```python
from build123d import *

# Parameters (mm, degrees)
CROQUIS1_R                = 1.5
SALIENTE_EXTRUIR1_DEPTH   = 10
SALIENTE_EXTRUIR1_2_DEPTH = 10
CROQUIS2_W                = 22.2
CROQUIS2_H                = 12
SALIENTE_EXTRUIR2_DEPTH   = 17.8
CROQUIS3_R                = 2.25
SALIENTE_EXTRUIR3_DEPTH   = 3
CROQUIS4_W                = 14.9
CROQUIS4_H                = 6.9
SALIENTE_EXTRUIR4_DEPTH   = 10
CROQUIS5_W                = 12.9
CROQUIS5_H                = 4.9
CROQUIS5_W_2              = 10.8
CROQUIS5_H_2              = 1.83
CORTAR_EXTRUIR1_DEPTH     = 10.5


with BuildPart() as part:
    # Croquis1 → Saliente-Extruir1 (new body)
    with BuildSketch(Plane.XY):
        with BuildLine():
            Line((-9.1, 6), (-9.1, -6))
            Line((-9.1, -6), (-13.25, -6))
            ThreePointArc((-13.25, -6), (-19.25, 0), (-13.25, 6))
            Line((-13.25, 6), (-9.1, 6))
        make_face()
        with Locations((-14.45, 0)):
            Circle(CROQUIS1_R, mode=Mode.SUBTRACT)
    extrude(amount=SALIENTE_EXTRUIR1_DEPTH)



with BuildPart() as body_2:
    # Croquis1 → Saliente-Extruir1 2 (new body)
    with BuildSketch(Plane.XY):
        with BuildLine():
            Line((9.1, 6), (9.1, -6))
            Line((9.1, -6), (13.25, -6))
            ThreePointArc((13.25, -6), (19.25, 0), (13.25, 6))
            Line((13.25, 6), (9.1, 6))
        make_face()
        with Locations((14.45, 0)):
            Circle(CROQUIS1_R, mode=Mode.SUBTRACT)
    extrude(amount=SALIENTE_EXTRUIR1_2_DEPTH)


with BuildPart() as part_1:
    add(part.part)

    add(body_2.part)  # Saliente-Extruir2 merges body 2
    # Croquis2 → Saliente-Extruir2 (add)
    with BuildSketch(Plane.XY.offset(10)):
        Rectangle(CROQUIS2_W, CROQUIS2_H)
    extrude(amount=SALIENTE_EXTRUIR2_DEPTH)

    # Croquis3 → Saliente-Extruir3 (add)
    with BuildSketch(Plane.XY.offset(27.8)):
        Circle(CROQUIS3_R)
    extrude(amount=SALIENTE_EXTRUIR3_DEPTH)

    # Croquis4 → Saliente-Extruir4 (add)
    with BuildSketch(Plane(origin=(0, 0, 10), x_dir=(-1, 0, 0), z_dir=(0, 0, -1))):
        Rectangle(CROQUIS4_W, CROQUIS4_H)
    extrude(amount=SALIENTE_EXTRUIR4_DEPTH)

    # Croquis5 → Cortar-Extruir1 (cut)
    with BuildSketch(Plane(origin=(0, 0, 0), x_dir=(-1, 0, 0), z_dir=(0, 0, -1))):
        Rectangle(CROQUIS5_W, CROQUIS5_H)
        with Locations((0, 0.915)):
            Rectangle(CROQUIS5_W_2, CROQUIS5_H_2, mode=Mode.SUBTRACT)
    extrude(amount=-CORTAR_EXTRUIR1_DEPTH, mode=Mode.SUBTRACT)


solid = part_1.part
```
Check sheet for the modelled part. Datum: model origin and axes. Units: mm. A direction names the side the tool comes from. Round coordinates to 2 decimals unless told otherwise and drop trailing zeros. Write each loop counter-clockwise with the first axis right and the second up, starting at its lowest first coordinate (ties: lowest second). Pieces come first, ordered by that corner, then holes. Notation, with made-up numbers: (73.5, 61) -> (128.5, 61) arc R13 cw to (128.5, 74) -> close; hole circle Ø3 at (87.25, 2). An arc over 180 degrees is marked (long way). Put each result on its own line as item: value.
(1) Material ranges on line 1 (Y direction, x = -5, z = 6); line 2 (X direction, y = -1.25, z = 8); line 3 (Z direction, x = -12.5, y = -0.5), recorded low to high.
Values found:
line 1: y = -3.45 to -2.45, 0 to 1.83, 2.45 to 3.45
line 2: x = -19.12 to -15.28, -13.62 to -9.1, -7.45 to -6.45, 6.45 to 7.45, 9.1 to 13.62, 15.28 to 19.12
line 3: z = 0 to 10
(2) Tool access check on faces 1 (the face through (-13, -1, 10)), 2 (the face through (0, 0, 30.8)), 3 (the face through (0, 1, 0)), 4 (the face through (0, 0, 5)), 5 (the face through (-9.1, 0, 5)). Record the directions out of +Z, -Z, +X, -X, +Y, -Y that give a thin tool (end or side, any length) a straight path to the whole face; none if there is none.
Values found:
face 1: +Z, -X, +Y, -Y
face 2: +Z, +X, -X, +Y, -Y
face 3: -Z, +X, -X, +Y, -Y
face 4: -Z
face 5: -Z, +Y, -Y
(3) Sectioned sample at D-D (x = 0). Enter the section's corners in (y, z).
Values found:
outline: (-6, 10) -> (-3.45, 10) -> (-3.45, 0) -> (-2.45, 0) -> (-2.45, 10.5) -> (0, 10.5) -> (0, 0) -> (1.83, 0) -> (1.83, 10.5) -> (2.45, 10.5) -> (2.45, 0) -> (3.45, 0) -> (3.45, 10) -> (6, 10) -> (6, 27.8) -> (2.25, 27.8) -> (2.25, 30.8) -> (-2.25, 30.8) -> (-2.25, 27.8) -> (-6, 27.8) -> close
(4) Sectioned sample at C-C (y = -3). Enter the section's corners in (x, z), plus the area to 3 significant figures.
Values found:
outline: (-18.45, 0) -> (-9.1, 0) -> (-9.1, 10) -> (-7.45, 10) -> (-7.45, 0) -> (7.45, 0) -> (7.45, 10) -> (9.1, 10) -> (9.1, 0) -> (18.45, 0) -> (18.45, 10) -> (11.1, 10) -> (11.1, 27.8) -> (-11.1, 27.8) -> (-11.1, 10) -> (-18.45, 10) -> close
area: 731 mm^2
(5) Sectioned sample at B-B (x = 14.45). Enter the section's corners in (y, z), plus the area to 3 significant figures.
Values found:
outline: (-5.88, 0) -> (-1.5, 0) -> (-1.5, 10) -> (-5.88, 10) -> close; (1.5, 0) -> (5.88, 0) -> (5.88, 10) -> (1.5, 10) -> close
area: 87.6 mm^2
(6) Mould release check, pull along X, two halves, no side actions. Record for faces 6 (the face through (6.45, 0, 5)), 7 (the face through (19.25, -0.13, 4.93)), 8 (the face through (-0.29, 2.23, 29.28)), 9 (the face through (13, -1, 10)): released by +X, released by -X, zero draft, split by the parting line, or undercut.
Values found:
face 6: undercut
face 7: released by +X
face 8: split by the parting line
face 9: zero draft
(7) Sectioned sample at A-A (z = 8). Enter the section's corners in (x, y).
Values found:
outline: (-13.25, -6) -> (-9.1, -6) -> (-9.1, 6) -> (-13.25, 6) arc R6 ccw to start; (-7.45, -3.45) -> (7.45, -3.45) -> (7.45, 3.45) -> (-7.45, 3.45) -> close; (-5.4, 0) -> (5.4, 0) -> (5.4, 1.83) -> (-5.4, 1.83) -> close; (9.1, -6) -> (13.25, -6) arc R6 ccw to (13.25, 6) -> (9.1, 6) -> close; hole circle Ø3 at (-14.45, 0); hole (-6.45, -2.45) -> (6.45, -2.45) -> (6.45, 2.45) -> (-6.45, 2.45) -> close; hole circle Ø3 at (14.45, 0)
(8) Go/stop test with flat-tipped pins: pin 1 Ø4 at (x, y) = (15.5, -0.5) entering from +Z; pin 2 Ø11 at (x, z) = (-1.5, 3) entering from +Y; pin 3 Ø8.5 at (x, z) = (-2, 4.5) entering from -Y. Record where each tip stops, or that it passes through.
Values found:
pin 1: stops at z = 10
pin 2: stops at y = 3.45
pin 3: stops at y = -3.45
